Read the model definition and answer for the solid it produces. Units are mm, in the model's axes. Face numbers are marked on the shaded views. A direction names the side the tool comes from. Coordinates: 2 decimals unless noted, no trailing zeros. Write each loop counter-clockwise with the first axis right and the second up, starting at its lowest first coordinate (ties: lowest second). Pieces come first, ordered by that corner, then holes.
(1) Determine the mould class of the marked faces 1, 2, 3 and 4 for opening direction Y: pulls with the +Y half, pulls with the -Y half, needs draft (parallel to the pull), parting line crosses it, or undercut.
(2) Which of the six approach directions +Z, -Z, +X, -X, +Y, -Y give full straight-line access (tool end or side, diameter ignored) to the marked faces 5, 6 and 7?
(3) Given pin 1 (1 mm diameter, centred on y = -3, z = 42, fed in from +X); pin 2 (11.5 mm diameter, centred on x = 44.5, y = -19, fed in from +Z); pin 3 (6.5 mm diameter, centred on y = -13.5, z = 8.5, fed in from +X), each flat-ended and moving along its own axis, determine where each tip first touches the part or whether it passes through.
(4) The part is cut by section C-C, the plane z = 16. Determine the outline of the cut face in (x, y) (3 decimals), and give its area (3 significant figures).
(5) Straight lines are drawn through the part: line 1 along Y through (x, z) = (42, 22); line 2 along Z through (x, y) = (40, 8); line 3 along X through (y, z) = (-38, 41). For each, find the intervals that lie inside material, in ascending order.
(6) The part is cut by section A-A, the plane x = 47. Determine the outline of the cut face in (y, z).
(7) The part is cut by section B-B, the plane y = -13. Determine the outline of the cut face in (x, z).
(8) The part is cut by section D-D, the plane y = -37.5. Determine the outline of the cut face in (x, z).
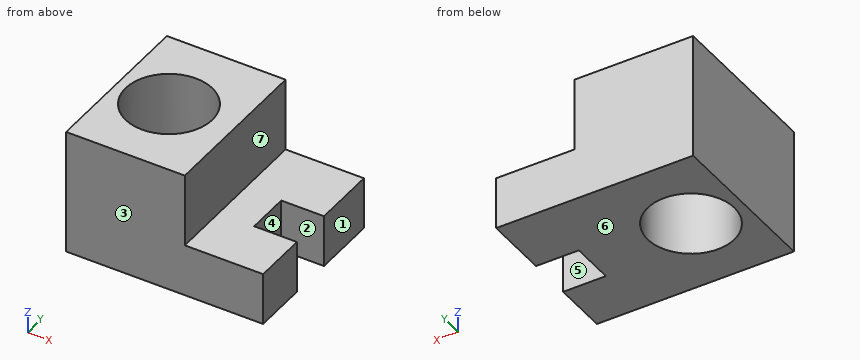
```python
from build123d import *

# Parameters (mm, degrees)
F0_W     = 95.312461257
F0_H     = 78.4068834037
F1_DEPTH = 25.4
F2_W     = 20.6947550178
F2_H     = 21.0718084127
F3_DEPTH = 25.4
F4_W     = 57.420656085
F4_H     = 78.4068834037
F5_DEPTH = 35.56
F8_D     = 41.91


with BuildPart() as f1:
    # F0 (on Top) → F1 (new body)
    with BuildSketch(Plane.XY):
        with Locations((12.0962299407, -8.1613110378)):
            Rectangle(F0_W, F0_H)
    extrude(amount=F1_DEPTH)

    # F2 (on face) → F3 (cut)
    with BuildSketch(Plane.XY.offset(25.4)):
        with Locations((49.4050830603, -10.5359042063)):
            Rectangle(F2_W, F2_H)
    extrude(amount=-F3_DEPTH, mode=Mode.SUBTRACT)

    # F4 (on face) → F5 (join)
    with BuildSketch(Plane.XY.offset(25.4)):
        with Locations((-6.8496726453, -8.1613110378)):
            Rectangle(F4_W, F4_H)
    extrude(amount=F5_DEPTH)

    # F8 (through all)
    with Locations(Plane.XY.offset(60.96)):
        with Locations((-9.9101644009, -8.5985241458)):
            Hole(F8_D / 2)


solid = f1.part
```
Computed:
1. face 1: needs draft
1. face 2: undercut
1. face 3: pulls with the -Y half
1. face 4: undercut
2. face 5: +Z, -Z, +X
2. face 6: -Z, +X, -X, +Y, -Y
2. face 7: +Z, +X, +Y, -Y
3. pin 1: stops at x = 21.86
3. pin 2: stops at z = 25.4
3. pin 3: stops at x = 39.06
4. outline: (-35.56, -47.365) - (59.752, -47.365) - (59.752, -21.072) - (39.058, -21.072) - (39.058, 0) - (59.752, 0) - (59.752, 31.042) - (-35.56, 31.042) - close; hole circle Ø41.91 at (-9.91, -8.599)
4. area: 5,660 mm2
5. line 1: y = -47.36 to -21.07, 0 to 31.04
5. line 2: z = 0 to 25.4
5. line 3: x = -35.56 to 21.86
6. outline: (-47.36, 0) - (-21.07, 0) - (-21.07, 25.4) - (-47.36, 25.4) - close; (0, 0) - (31.04, 0) - (31.04, 25.4) - (0, 25.4) - close
7. outline: (-35.56, 0) - (-30.4, 0) - (-30.4, 60.96) - (-35.56, 60.96) - close; (10.58, 0) - (39.06, 0) - (39.06, 25.4) - (21.86, 25.4) - (21.86, 60.96) - (10.58, 60.96) - close
8. outline: (-35.56, 0) - (59.75, 0) - (59.75, 25.4) - (21.86, 25.4) - (21.86, 60.96) - (-35.56, 60.96) - close
